from build123d import *

# Parameters (mm, degrees)
BOSS_EXTRUDE1_DEPTH                                  = 76.2
CBORE_FOR_1_4_BINDING_HEAD_MACHINE_SCREW_D           = 6.7564
CBORE_FOR_1_4_BINDING_HEAD_MACHINE_SCREW_CBORE_D     = 14.2875
CBORE_FOR_1_4_BINDING_HEAD_MACHINE_SCREW_CBORE_DEPTH = 54.991


with BuildPart() as part:
    # Sketch1 → Boss-Extrude1 (new body)
    with BuildSketch(Plane(origin=(0, 0, 0), x_dir=(1, 0, 0), z_dir=(0, 1, 0))):
        Polygon((0, -7.505553499), (6.5, -3.75277675), (6.5, 3.75277675), (6.5, 12.7), (31.75, 12.7), (31.75, -12.7), (-31.75, -12.7), (-31.75, 12.7), (-6.5, 12.7), (-6.5, 3.75277675), (-6.5, -3.75277675), align=None)
    extrude(amount=BOSS_EXTRUDE1_DEPTH)

    # CBORE for 1/4 Binding Head Machine Screw1 (through all)
    with Locations(Plane(origin=(0, 76.2, 0), x_dir=(1, 0, 0), z_dir=(0, 1, 0))):
        with Locations((-19.125, 0), (19.125, 0)):
            CounterBoreHole(CBORE_FOR_1_4_BINDING_HEAD_MACHINE_SCREW_D / 2, CBORE_FOR_1_4_BINDING_HEAD_MACHINE_SCREW_CBORE_D / 2, CBORE_FOR_1_4_BINDING_HEAD_MACHINE_SCREW_CBORE_DEPTH)


solid = part.part
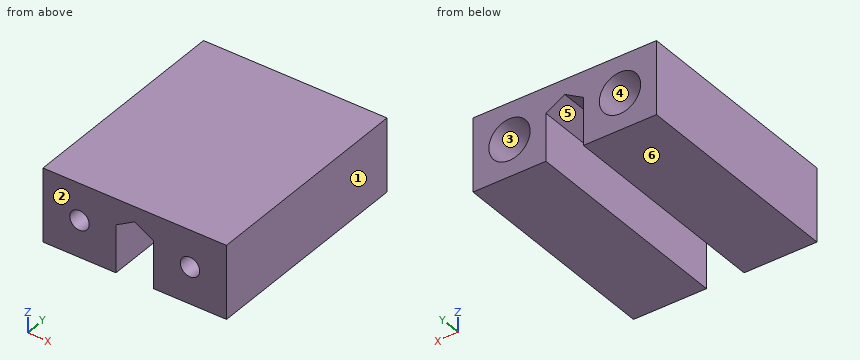
Design review of the part built by this model. Coordinates are the model's own, in mm. Face numbers are marked on the shaded views. A direction names the side the tool comes from. Round coordinates to 2 decimals unless told otherwise and drop trailing zeros. Loops run counter-clockwise (first coordinate to the right, second up) from the corner with the lowest first, then second, coordinate; pieces in that order, holes last. Notation, with made-up numbers: M -4,64.25 L 33,64.25 A18 ccw 33,85.25 Z; hole C -21.75,69 d1. An arc over 180 degrees is marked long. Answer as a JSON object with one key per item and string values.
Item 1: Wall thickness on L1, parallel to Z at x = 19, y = 21.5; L2, parallel to X at y = 61, z = 1.25; L3, parallel to Z at x = 16.5, y = 59: over which ranges is each line inside the solid? List them lowest first. Write a range as from..to.
Answer sheet:
{"L1": "z = -12.7..-7.14, 7.14..12.7", "L2": "x = -31.75..-26.16, -12.09..-6.5, 6.5..12.09, 26.16..31.75", "L3": "z = -12.7..-6.64, 6.64..12.7"}
Item 2: The part is to be moulded in two halves that separate along X. For the marked faces 1, 2 and 3, say which applies: pulls with the +X half, pulls with the -X half, needs draft (parallel to the pull), parting line crosses it, or undercut.
Answer sheet:
{"face 1": "pulls with the +X half", "face 2": "needs draft", "face 3": "undercut"}
Item 3: We need section C-C on z = -6.25. Give the boundary of the cut face in (x, y), and give its area (3 significant figures).
Answer sheet:
{"outline": "M -31.75,0 L -6.5,0 L -6.5,76.2 L -15.67,76.2 L -15.67,21.21 L -22.58,21.21 L -22.58,76.2 L -31.75,76.2 Z; M 6.5,0 L 31.75,0 L 31.75,76.2 L 22.58,76.2 L 22.58,21.21 L 15.67,21.21 L 15.67,76.2 L 6.5,76.2 Z", "area": "3,090 mm^2"}
Item 4: Machinability: for the marked faces 4, 5 and 6, which of the approach directions +Z, -Z, +X, -X, +Y, -Y give a long, thin tool a straight path to every point of the face, cutting with its end or side? Answer none if there is none.
Answer sheet:
{"face 4": "+Y", "face 5": "-Z, +Y, -Y", "face 6": "-Z, +X, -X, +Y, -Y"}
Item 5: We need section B-B on y = 60.5. State how many separate pieces and enclosed holes the cut face has, and give its area (3 significant figures).
Answer sheet:
{"separate pieces": "1", "enclosed holes": "2", "area": "1,050 mm^2"}
Item 6: Clearance check with a flat-ended pin moving along its axis: P1, Ø9, axis at x = 19.125, z = 0, coming from the +Y side. State where the tip first meets the part, or that it passes through.
Answer sheet:
{"P1": "stops at y = 21.21"}
Item 7: We need section A-A on z = 0. Give the boundary of the cut face in (x, y), and give its area (3 significant figures).
Answer sheet:
{"outline": "M -31.75,0 L -22.5,0 L -22.5,21.21 L -26.27,21.21 L -26.27,76.2 L -31.75,76.2 Z; M -15.75,0 L -6.5,0 L -6.5,76.2 L -11.98,76.2 L -11.98,21.21 L -15.75,21.21 Z; M 6.5,0 L 15.75,0 L 15.75,21.21 L 11.98,21.21 L 11.98,76.2 L 6.5,76.2 Z; M 22.5,0 L 31.75,0 L 31.75,76.2 L 26.27,76.2 L 26.27,21.21 L 22.5,21.21 Z", "area": "1,990 mm^2"}
Item 8: We need section D-D on x = -14. Give the boundary of the cut face in (y, z), and give its area (3 significant figures).
Answer sheet:
{"outline": "M 0,-12.7 L 76.2,-12.7 L 76.2,-4.98 L 21.21,-4.98 L 21.21,4.98 L 76.2,4.98 L 76.2,12.7 L 0,12.7 Z", "area": "1,390 mm^2"}
